Build history of the part. All positions in model axes, mm. A direction names the side the tool comes from. Round coordinates to 2 decimals unless told otherwise and drop trailing zeros. Loops run counter-clockwise (first coordinate to the right, second up) from the corner with the lowest first, then second, coordinate; pieces in that order, holes last. Notation, with made-up numbers: (-36.5, 52.5) - (-1.5, 52.5) arc R19 ccw to (-1.5, 67.5) - close; hole circle Ø10 at (52, 4.25). An arc over 180 degrees is marked (long way). Answer as CSV lines item,"result". Start each with the question number.
```python
from build123d import *

# Parameters (mm, degrees)
F0_R     = 2
F1_DEPTH = 3


with BuildPart() as f1:
    # F0 (on Front) → F1 (new body)
    with BuildSketch(Plane.XZ):
        with BuildLine():
            Line((4.503332, 0), (2.251666, -3.9))
            Line((2.251666, -3.9), (-2.251666, -3.9))
            Line((-2.251666, -3.9), (-2.251666, -5.4))
            ThreePointArc((-2.251666, -5.4), (3.104614, -7.981328), (8.762644, -6.153846))
            ThreePointArc((8.762644, -6.153846), (10.259084, -5.2973), (11.9575, -5))
            Line((11.9575, -5), (75, -5))
            ThreePointArc((75, -5), (80, 0), (75, 5))
            Line((75, 5), (11.9575, 5))
            ThreePointArc((11.9575, 5), (10.259084, 5.2973), (8.762644, 6.153846))
            ThreePointArc((8.762644, 6.153846), (3.104614, 7.981328), (-2.251666, 5.4))
            Line((-2.251666, 5.4), (-2.251666, 3.9))
            Line((-2.251666, 3.9), (2.251666, 3.9))
            Line((2.251666, 3.9), (4.503332, 0))
        make_face()
        with Locations((75, 0)):
            Circle(F0_R, mode=Mode.SUBTRACT)
    extrude(amount=F1_DEPTH)


solid = f1.part
```
Q1. Tool access for faces 1 (the flat face through (-2.252, -1, 5)), 2 (the flat face through (3.36, -1.48, 1.98)), 3 (the flat face through (44, -1, 5)), 4 (the flat face through (43, -1, -5)), 5 (the cylindrical face through (3.19, -1.479, 7.987)): list every direction of +Z, -Z, +X, -X, +Y, -Y with a clear straight run to the whole face (end or side of a thin tool).
Q2. Band-saw the part on B-B, the plane x = 27. List the corners of the cut face in (y, z), then the cut area to 3 significant figures.
Q3. Two-plate mould, pull along Z, no slides. Class faces 6 (the flat face through (38, -3, 0)), 7 (the cylindrical face through (10.236, -1.479, -5.306)), 8 (the flat face through (3.393, -1.479, -1.923)): released by +Z, released by -Z, zero draft, split by the parting line, or undercut.
Q4. Band-saw the part on A-A, the plane y = -1.9. List the corners of the cut face in (x, z).
Q5. Pin check, flat tip, straight feed: pin 1 Ø1.5 at (x, y) = (0, -1.5) entering from +Z. Stop position of the tip, or through.
Q6. Wall check: probe 1 along Z at (x, y) = (75, -1.2); probe 2 along Z at (x, y) = (71, -2.55); probe 3 along X at (y, z) = (-0.4, 1.25). Give the ranges that are in metal, low to high. Write a range as [from, to].
Reported:
1,face 1,"+Z, -Z, -X, +Y, -Y"
1,face 2,"-X, +Y, -Y"
1,face 3,"+Z, +X, +Y, -Y"
1,face 4,"-Z, +X, +Y, -Y"
1,face 5,"+Z, +Y, -Y"
2,outline,"(-3, -5) - (0, -5) - (0, 5) - (-3, 5) - close"
2,area,"30.0 mm2"
3,face 6,"zero draft"
3,face 7,"released by -Z"
3,face 8,"undercut"
4,outline,"(-2.25, -5.4) arc R8 ccw to (8.76, -6.15) arc R5 cw to (11.96, -5) - (75, -5) arc R5 ccw to (75, 5) - (11.96, 5) arc R5 cw to (8.76, 6.15) arc R8 ccw to (-2.25, 5.4) - (-2.25, 3.9) - (2.25, 3.9) - (4.5, 0) - (2.25, -3.9) - (-2.25, -3.9) - close; hole circle Ø4 at (75, 0)"
5,pin 1,"stops at z = 7.46"
6,probe 1,"z = [-5, -2], [2, 5]"
6,probe 2,"z = [-5, 5]"
6,probe 3,"x = [3.78, 73.44], [76.56, 79.84]"
